Here's the drawing with two shaded views (mm, measured from the low corner). I have some questions. A direction names the side the tool comes from. Round coordinates to 2 decimals unless told otherwise and drop trailing zeros. Loops run counter-clockwise (first coordinate to the right, second up) from the corner with the lowest first, then second, coordinate; pieces in that order, holes last. Notation, with made-up numbers: (-6, -33.75) -> (2, -33.75) arc R21 ccw to (2, -19.75) -> close; hole circle Ø5 at (39, 7). An arc over 180 degrees is marked (long way). Write each question's results on one line, items separated by ' | '. Start each with the question number.
1) For P1, Ø6, axis at x = 54, z = 16, coming from the -Y side; P2, Ø5.5, axis at y = 9, z = 23.5, coming from the -X side; P3, Ø9, axis at y = 8.5, z = 18.5, coming from the +X side; P4, Ø2.5, axis at x = 5, z = 5, coming from the +Y side, each with a flat end and sliding along its axis, tell me the tip position at first contact or that it passes through.
2) We'd pull the mould along Z, two halves only. Please class the marked faces 1, 2 and 3: pulls with the +Z half, pulls with the -Z half, needs draft (parallel to the pull), parting line crosses it, or undercut.
3) If I drill on probe 1 along X at (y, z) = (1.25, 35); probe 2 along Z at (x, y) = (65, 2.2); probe 3 along X at (y, z) = (20, 13.5), over which ranges is the centre line in solid material (lowest first)?
4) Imagine slicing it at A-A, the plane y = 11. List the corners of the cut face in (x, z) for me, plus the area to 3 significant figures.
5) Imagine slicing it at B-B, the plane z = 35. List the corners of the cut face in (x, y) for me, plus the area to 3 significant figures.
6) Which directions (+Z, -Z, +X, -X, +Y, -Y) give clear straight access to the entire face, cutting with the end or side of a thin tool? Please do the marked faces 4, 5, 6, 7 and 8.
7) Imagine slicing it at C-C, the plane x = 57. List the corners of the cut face in (y, z) for me.
8) Imagine slicing it at D-D, the plane y = 21. List the corners of the cut face in (x, z) for me, plus the area to 3 significant figures.
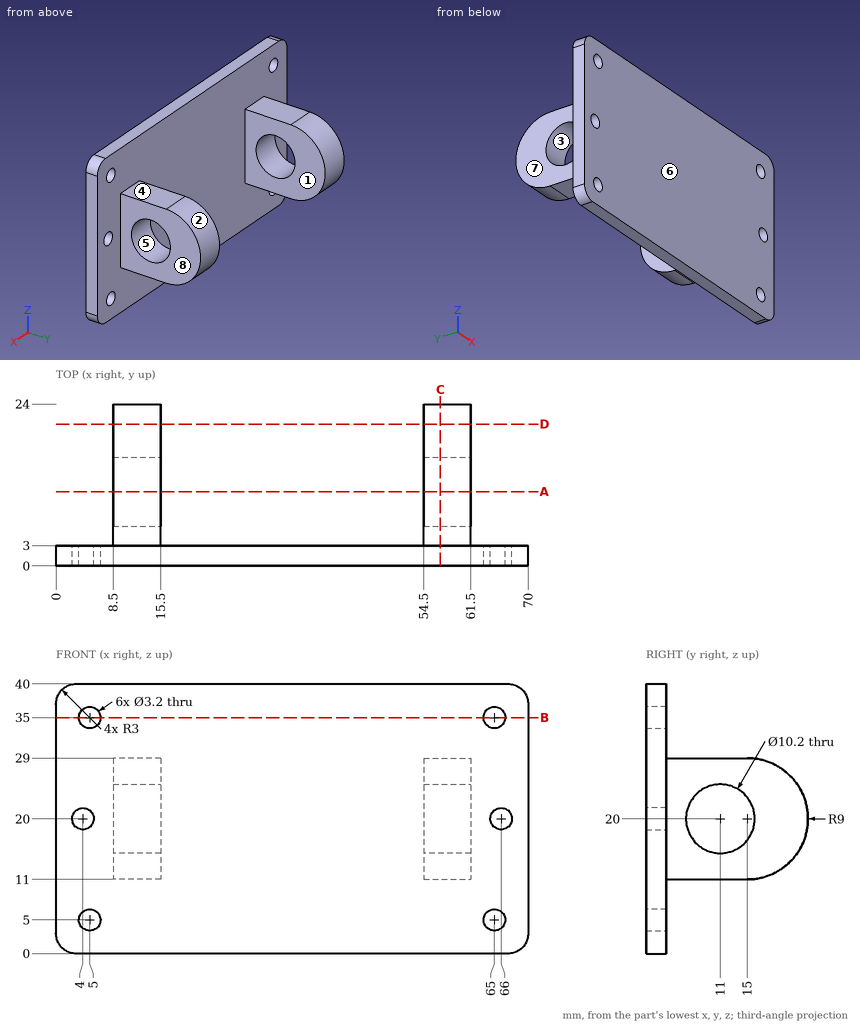
Checked values:
1) P1: y = 0 | P2: x = 8.5 | P3: x = 61.5 | P4: through
2) face 1: needs draft | face 2: parting line crosses it | face 3: undercut
3) probe 1: 0 to 3.4, 6.6 to 63.4, 66.6 to 70 | probe 2: 0 to 3.4, 6.6 to 18.75, 21.25 to 33.4, 36.6 to 40 | probe 3: 8.5 to 15.5, 54.5 to 61.5
4) outline: (8.5, 11) -> (15.5, 11) -> (15.5, 14.9) -> (8.5, 14.9) -> close; (8.5, 25.1) -> (15.5, 25.1) -> (15.5, 29) -> (8.5, 29) -> close; (54.5, 11) -> (61.5, 11) -> (61.5, 14.9) -> (54.5, 14.9) -> close; (54.5, 25.1) -> (61.5, 25.1) -> (61.5, 29) -> (54.5, 29) -> close | area: 109 mm^2
5) outline: (0, 0) -> (3.4, 0) -> (3.4, 3) -> (0, 3) -> close; (6.6, 0) -> (63.4, 0) -> (63.4, 3) -> (6.6, 3) -> close; (66.6, 0) -> (70, 0) -> (70, 3) -> (66.6, 3) -> close | area: 191 mm^2
6) face 4: +Z, +X, -X, +Y | face 5: +X, -X | face 6: +Z, -Z, +X, -X, -Y | face 7: +Z, -Z, -X, +Y | face 8: +Z, -Z, +X, +Y
7) outline: (0, 0) -> (3, 0) -> (3, 11) -> (15, 11) arc R9 ccw to (15, 29) -> (3, 29) -> (3, 40) -> (0, 40) -> close; hole circle Ø10.2 at (11, 20)
8) outline: (8.5, 13.29) -> (15.5, 13.29) -> (15.5, 26.71) -> (8.5, 26.71) -> close; (54.5, 13.29) -> (61.5, 13.29) -> (61.5, 26.71) -> (54.5, 26.71) -> close | area: 188 mm^2
